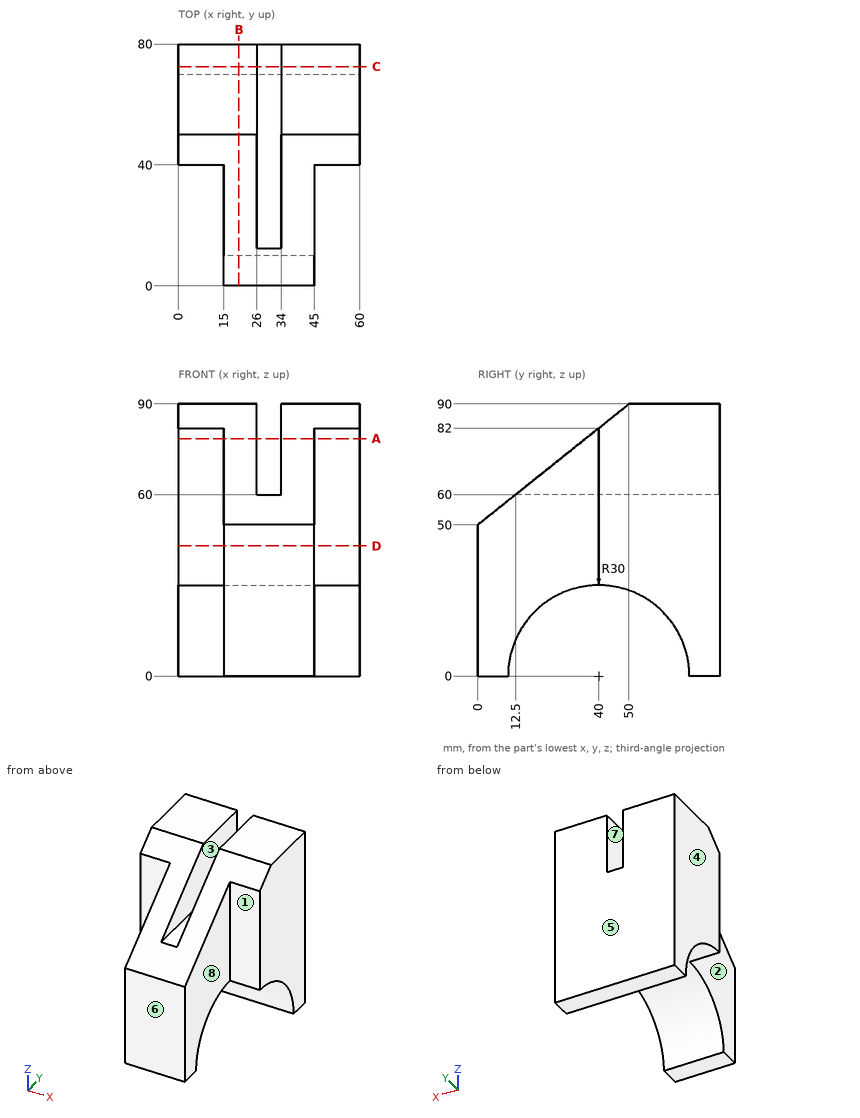
Geometry: see drawing. Coordinates: mm, zero at the bounding-box minimum. A direction names the side the tool comes from. Coordinates: 2 decimals unless noted, no trailing zeros. Loops run counter-clockwise (first coordinate to the right, second up) from the corner with the lowest first, then second, coordinate; pieces in that order, holes last.
(1) Section C-C on y = 72.5. Return the cut outline in (x, z).
(2) Pull-direction query (X, two-part tool) for the marked faces 6, 7 and 8; classes: released by +X, released by -X, zero draft, split by the parting line, or undercut.
(3) Material intervals for probe 1 along Y at (x, z) = (48.5, 41.5); probe 2 along X at (y, z) = (49, 66.5); probe 3 along X at (y, z) = (14, 57.5), sorted ascending.
(4) Section B-B on x = 20. Return the cut outline in (y, z), then the cut area to 3 significant figures.
(5) Section D-D on z = 43. Return the cut outline in (x, y).
(6) First-contact query: pin 1 Ø4.5 at (x, z) = (55.5, 54.5) entering from -Y; pin 2 Ø15 at (y, z) = (29.5, 71) entering from -X; pin 3 Ø1 at (x, y) = (25.5, 16) entering from +Z; pin 4 Ø10 at (y, z) = (22.5, 17.5) entering from -X. Flat tips, straight axial feed; report the tip coordinate or a pass-through.
(7) Section A-A on z = 78.5. Return the cut outline in (x, y) (3 decimals), then the cut area to 3 significant figures.
(8) Set-up query: the marked faces 1, 2, 3, 4 and 5. Return all of +Z, -Z, +X, -X, +Y, -Y with unobstructed straight access to the full face (end or side cutting, diameter ignored); none if empty.
Data:
1. outline: (0, 0) - (60, 0) - (60, 90) - (34, 90) - (34, 60) - (26, 60) - (26, 90) - (0, 90) - close
2. face 6: zero draft
2. face 7: undercut
2. face 8: released by +X
3. probe 1: y = 40 to 80
3. probe 2: x = 0 to 26, 34 to 60
3. probe 3: x = 15 to 45
4. outline: (0, 0) - (10, 0) arc R30 cw to (70, 0) - (80, 0) - (80, 90) - (50, 90) - (0, 50) - close
4. area: 4,790 mm2
5. outline: (0, 40) - (15, 40) - (15, 0) - (45, 0) - (45, 40) - (60, 40) - (60, 80) - (0, 80) - close
6. pin 1: stops at y = 40
6. pin 2: stops at x = 15
6. pin 3: stops at z = 63.2
6. pin 4: passes through
7. outline: (0, 40) - (15, 40) - (15, 35.625) - (26, 35.625) - (26, 80) - (0, 80) - close; (34, 35.625) - (45, 35.625) - (45, 40) - (60, 40) - (60, 80) - (34, 80) - close
7. area: 2,180 mm2
8. face 1: +Z, -Z, +X, -Y
8. face 2: +Z, -Z, -X, -Y
8. face 3: +Z, +Y, -Y
8. face 4: +Z, -Z, -X, +Y, -Y
8. face 5: +Z, -Z, +X, -X, +Y
